The listing builds one solid part. Answer for the finished solid, in the listing's coordinates (mm). A direction names the side the tool comes from. Coordinates: 2 decimals unless noted, no trailing zeros. Loops run counter-clockwise (first coordinate to the right, second up) from the corner with the lowest first, then second, coordinate; pieces in that order, holes last. Notation, with made-up numbers: M 17,85 L 64,85 A21 cw 64,119 Z; hole C 48.5,42.25 d9. An arc over 180 degrees is marked long. Answer as a JSON object with one key per item and string values. Group by question number.
1. Straight lines are drawn through the part: L1, parallel to Y at x = 0.25, z = 30.5; L2, parallel to X at y = -0.25, z = 16. For each, find the intervals that lie inside material, in ascending order.
2. Given pin 1 (8 mm diameter, centred on x = -1.5, y = -1.5, fed in from -Z); pin 2 (4 mm diameter, centred on y = 3.5, z = 17.5, fed in from -X); pin 3 (4.5 mm diameter, centred on y = 1, z = 32, fed in from -X); pin 4 (6 mm diameter, centred on y = -5, z = 18, fed in from -X), each flat-ended and moving along its own axis, determine where each tip first touches the part or whether it passes through.
3. A cutting plane is placed at C-C on z = 31. Give the vertices of the cut face in (x, y), and give its area (3 significant figures).
4. A cutting plane is placed at D-D on z = 22. Give the vertices of the cut face in (x, y), and give its area (3 significant figures).
5. For faces 1 (the face through (0, 5.5, 31)), 2 (the face through (4.93, 4.9, 31.33)), 3 (the face through (-4, 5, 22.9)), 4 (the face through (0, -5.5, 31)), determine the directions among +Z, -Z, +X, -X, +Y, -Y from which every point of the face is accessible in a straight line to the end or side of a thin tool.
6. A cutting plane is placed at A-A on x = 0. Give the vertices of the cut face in (y, z).
Autodesk Inventor part; units mm, degrees
ref_plane "YZ Plane" through (0, 0, 0) normal (1, 0, 0) x (0, 1, 0)
ref_plane "XZ Plane" through (0, 0, 0) normal (0, 1, 0) x (-1, 0, 0)
ref_plane "XY Plane" through (0, 0, 0) normal (0, 0, 1) x (1, 0, 0)
sketch "Sketch1" plane through (0, 0, 0) normal (0, 0, 1) x (1, 0, 0)
  circle A0 centre (0, 0) radius 6
  dimension "d0" = 12
extrude "Extrusion1" add sketch "Sketch1" along normal blind 22.9
sketch "Sketch2" plane through (0, 0, 22.9) normal (0, 0, 1) x (1, 0, 0)
  line L0 (-7.75, 7.75) -> (7.75, 7.75)
  line L1 (7.75, 7.75) -> (7.75, -7.75)
  line L2 (7.75, -7.75) -> (-7.75, -7.75)
  line L3 (-7.75, -7.75) -> (-7.75, 7.75)
  line L4 (-7.75, 7.75) -> (7.75, -7.75) construction
  line L5 (7.75, 7.75) -> (-7.75, -7.75) construction
  point P0 (0, 0)
  dimension "d3" = 15.5
  dimension "d4" = 15.5
extrude "Extrusion2" add sketch "Sketch2" along normal blind 6.4
sketch "Sketch3" plane through (0, 0, 29.3) normal (0, 0, 1) x (1, 0, 0)
  line L0 (-5.5, 5.5) -> (5.5, 5.5)
  line L1 (5.5, 5.5) -> (5.5, -5.5)
  line L2 (5.5, -5.5) -> (-5.5, -5.5)
  line L3 (-5.5, -5.5) -> (-5.5, 5.5)
  line L4 (-5.5, 5.5) -> (5.5, -5.5) construction
  line L5 (5.5, 5.5) -> (-5.5, -5.5) construction
  point P0 (0, 0)
  dimension "d7" = 11
  dimension "d8" = 11
extrude "Extrusion3" add sketch "Sketch3" along normal blind 6
fillet "Fillet1" radius 2 12 edges at (0, 5.5, 35.3) (5.5, 5.5, 32.3) (5.5, 0, 35.3) (0, -5.5, 35.3) (5.5, -5.5, 32.3) (-5.5, 0, 35.3) (-5.5, 5.5, 32.3) (-5.5, -5.5, 32.3) (-7.75, 0, 29.3) (0, -7.75, 29.3) (7.75, 0, 29.3) (0, 7.75, 29.3)
fillet "Fillet2" radius 2 8 edges at (7.1642, -7.1642, 28.7142) (7.75, -7.75, 25.1) (-7.1642, -7.1642, 28.7142) (-7.75, -7.75, 25.1) (7.1642, 7.1642, 28.7142) (7.75, 7.75, 25.1) (-7.1642, 7.1642, 28.7142) (-7.75, 7.75, 25.1)
properties part number "Power Switch"
From the geometry:
{
 "1": {"L1": "y = -5.5 to 5.5", "L2": "x = -5.99 to 5.99"},
 "2": {"pin 1": "stops at z = 0", "pin 2": "stops at x = -5.81", "pin 3": "stops at x = -5.5", "pin 4": "stops at x = -5.66"},
 "3": {"outline": "M -5.5,-3.5 A2 ccw -3.5,-5.5 L 3.5,-5.5 A2 ccw 5.5,-3.5 L 5.5,3.5 A2 ccw 3.5,5.5 L -3.5,5.5 A2 ccw -5.5,3.5 Z", "area": "118 mm²"},
 "4": {"outline": "C 0,0 d12", "area": "113 mm²"},
 "5": {"face 1": "+Z, +X, -X, +Y", "face 2": "+Z, +X, +Y", "face 3": "-Z", "face 4": "+Z, +X, -X, -Y"},
 "6": {"outline": "M -7.75,22.9 L -6,22.9 L -6,0 L 6,0 L 6,22.9 L 7.75,22.9 L 7.75,27.3 A2 ccw 5.75,29.3 L 5.5,29.3 L 5.5,33.3 A2 ccw 3.5,35.3 L -3.5,35.3 A2 ccw -5.5,33.3 L -5.5,29.3 L -5.75,29.3 A2 ccw -7.75,27.3 Z"}
}
